Geometry: see drawing. Coordinates: mm, zero at the bounding-box minimum. Coordinates: 2 decimals unless noted, no trailing zeros. Loops run counter-clockwise (first coordinate to the right, second up) from the corner with the lowest first, then second, coordinate; pieces in that order, holes last.
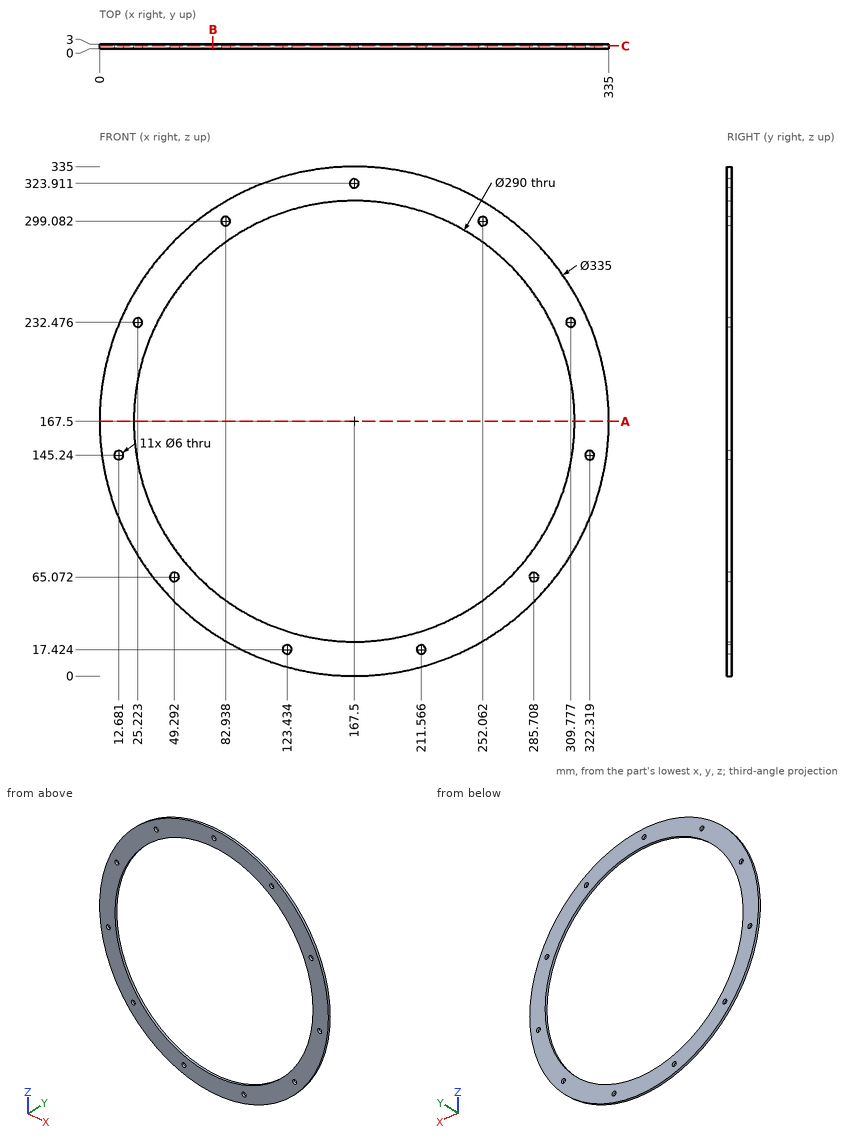
Item 1: Contact query for a flat-ended pin moving along its axis: P1, Ø5, axis at x = 167.5, z = 323.91, coming from the -Y side. Output: stop coordinate, or through.
Result:
P1: passes through
Item 2: Line query: L1, parallel to Z at x = 167.5, y = 1.3; L2, parallel to Z at x = 274.5, y = 0.2 (1 decimal); L3, parallel to X at y = 0.6, z = 183.5 (1 decimal). Output: solid intervals per line, ascending.
Result:
L1: z = 0 to 22.5, 312.5 to 320.91, 326.91 to 335
L2: z = 38.6 to 69.6, 265.4 to 296.4
L3: x = 0.8 to 23.4, 311.6 to 334.2
Item 3: Section query A-A (z = 167.5). Output: boundary loops of the cut face in (x, y).
Result:
outline: (0, 0) - (22.5, 0) - (22.5, 3) - (0, 3) - close; (312.5, 0) - (335, 0) - (335, 3) - (312.5, 3) - close
Item 4: Section query B-B (x = 74.5). Output: boundary loops of the cut face in (y, z).
Result:
outline: (0, 28.19) - (3, 28.19) - (3, 56.25) - (0, 56.25) - close; (0, 278.75) - (3, 278.75) - (3, 306.81) - (0, 306.81) - close
Item 5: Section query C-C (y = 1.8). Count the separate pieces of the cut face and the enclosed holes in it, then the cut area to 3 significant figures.
Result:
separate pieces: 1
enclosed holes: 12
area: 21,800 mm2
